Could you check a few things on this model? Use its own coordinates, in mm. Coordinates: 2 decimals unless noted, no trailing zeros. Loops run counter-clockwise (first coordinate to the right, second up) from the corner with the lowest first, then second, coordinate; pieces in that order, holes last.
1) Imagine slicing it at D-D on y = -21.5. Please give me the cut outline in (x, z), plus the area to 3 significant figures.
2) Will these pins go through, and if not, where does the flat tip stop? P1, Ø1, axis at x = 28, z = 2, coming from the -Y side; P2, Ø1.5, axis at x = 16.5, z = 2, coming from the -Y side.
3) Imagine slicing it at B-B on y = 0. Please give me the cut outline in (x, z), plus the area to 3 significant figures.
4) Imagine slicing it at A-A on z = 0.95. Please give me the cut outline in (x, y).
5) If I drill on line 1 along Y through (x, z) = (0, 0.8); line 2 along X through (y, z) = (-0.5, 0.95), over which ranges is the centre line in solid material (lowest first)?
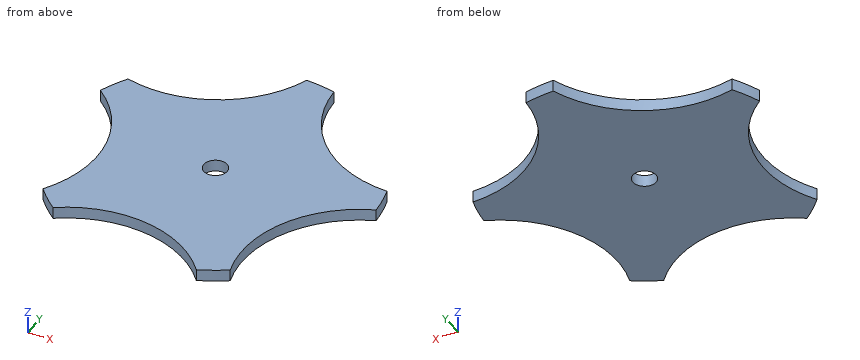
Autodesk Inventor part; units mm, degrees
ref_plane "YZ Plane" through (0, 0, 0) normal (1, 0, 0) x (0, 1, 0)
ref_plane "XZ Plane" through (0, 0, 0) normal (0, 1, 0) x (-1, 0, 0)
ref_plane "XY Plane" through (0, 0, 0) normal (0, 0, 1) x (1, 0, 0)
sketch "Sketch1" plane through (0, 0, 0) normal (0, 0, 1) x (1, 0, 0)
  circle A0 centre (0, 0) radius 40
  dimension "d0" = 80
extrude "Extrusion1" add sketch "Sketch1" along normal blind 3
sketch "Sketch2" plane through (0, 0, 3) normal (0, 0, 1) x (1, 0, 0)
  circle A0 centre (0, 0) radius 40
  circle A1 centre (40, 40) radius 30
  dimension "d6" = 60
  dimension "d7" = 40
  dimension "d8" = 40
extrude "Extrusion2" cut sketch "Sketch2" against normal through all contours A1 A0 | A0 A1 picked at (25.0118, 25.0118) picked at (39.5025, 38.7873)
pattern_circular "Circular Pattern1" count 5 over 360 about axis through (0, 0, -10) along (0, 0, 1) of "Extrusion2"
sketch "Sketch3" plane through (0, 0, 3) normal (0, 0, 1) x (1, 0, 0)
  point P0 (0, 0)
  point P1 (0, 0)
hole "Hole1" at (0, 0, 3) direction (0, 0, -1) diameter 6 end through all
properties part number "Pancake_Star" material "PC/ABS Plastic"
Filled in:
1. outline: (-28.67, 0) - (20.7, 0) - (20.7, 3) - (-28.67, 3) - close
1. area: 148 mm2
2. P1: stops at y = -6.3
2. P2: stops at y = -36.77
3. outline: (-27.21, 0) - (-3, 0) - (-3, 3) - (-27.21, 3) - close; (3, 0) - (34.9, 0) - (34.9, 3) - (3, 3) - close
3. area: 168 mm2
4. outline: (-37.22, 14.65) arc R30 cw to (-30.87, -25.43) arc R40 ccw to (-25.43, -30.87) arc R30 cw to (14.65, -37.22) arc R40 ccw to (21.5, -33.73) arc R30 cw to (39.93, 2.43) arc R40 ccw to (38.72, 10.03) arc R30 cw to (10.03, 38.72) arc R40 ccw to (2.43, 39.93) arc R30 cw to (-33.73, 21.5) arc R40 ccw to start; hole circle Ø6 at (0, 0)
5. line 1: y = -27.21 to -3, 3 to 34.9
5. line 2: x = -27.06 to -2.96, 2.96 to 34.1
